```python
from build123d import *

# Parameters (mm, degrees)
F1_DEPTH = 25


with BuildPart() as f1:
    # F0 (on Top) → F1 (new body)
    with BuildSketch(Plane.XY):
        with BuildLine():
            ThreePointArc((-35.28226, -29.26819), (-33.817794, -32.803724), (-30.28226, -34.26819))
            Line((-30.28226, -34.26819), (29.71774, -34.26819))
            ThreePointArc((29.71774, -34.26819), (33.253274, -32.803724), (34.71774, -29.26819))
            Line((34.71774, -29.26819), (34.71774, -8.26819))
            ThreePointArc((34.71774, -8.26819), (31.788808, -1.197122), (24.71774, 1.73181))
            Line((24.71774, 1.73181), (-25.28226, 1.73181))
            ThreePointArc((-25.28226, 1.73181), (-32.353327, -1.197122), (-35.28226, -8.26819))
            Line((-35.28226, -8.26819), (-35.28226, -29.26819))
        make_face()
        with BuildLine():
            ThreePointArc((-16.084487, -11.432007), (-15.556147, -11.258388), (-15.011794, -11.144518))
            Line((-15.011794, -11.144518), (-15.011794, -6.116113))
            ThreePointArc((-15.011794, -6.116113), (-14.261794, -6.087948), (-13.511794, -6.116113))
            Line((-13.511794, -6.116113), (-13.511794, -11.144518))
            ThreePointArc((-13.511794, -11.144518), (-12.967699, -11.258319), (-12.439598, -11.431812))
            Line((-12.439598, -11.431812), (-9.924919, -7.077315))
            ThreePointArc((-9.924919, -7.077315), (-9.59007, -7.246285), (-9.261794, -7.427694))
            ThreePointArc((-9.261794, -7.427694), (-8.940551, -7.621285), (-8.626794, -7.826787))
            Line((-8.626794, -7.826787), (-11.140977, -12.181479))
            ThreePointArc((-11.140977, -12.181479), (-10.72626, -12.552414), (-10.355325, -12.967131))
            Line((-10.355325, -12.967131), (-6.000633, -10.452948))
            ThreePointArc((-6.000633, -10.452948), (-5.60154, -11.087948), (-5.251161, -11.751073))
            Line((-5.251161, -11.751073), (-9.605852, -14.265255))
            ThreePointArc((-9.605852, -14.265255), (-9.432234, -14.793595), (-9.318364, -15.337948))
            Line((-9.318364, -15.337948), (-4.289958, -15.337948))
            ThreePointArc((-4.289958, -15.337948), (-4.261794, -16.087948), (-4.289958, -16.837948))
            Line((-4.289958, -16.837948), (-9.318364, -16.837948))
            ThreePointArc((-9.318364, -16.837948), (-9.432235, -17.382306), (-9.605856, -17.91065))
            Line((-9.605856, -17.91065), (-5.251199, -20.424903))
            Line((-5.251199, -20.424903), (-6.000683, -21.723021))
            Line((-6.000683, -21.723021), (-10.355352, -19.2088))
            ThreePointArc((-10.355352, -19.2088), (-10.726087, -19.623309), (-11.14056, -19.994084))
            Line((-11.14056, -19.994084), (-8.626357, -24.348811))
            ThreePointArc((-8.626357, -24.348811), (-9.261794, -24.748202), (-9.925395, -25.098811))
            Line((-9.925395, -25.098811), (-12.439598, -20.744084))
            ThreePointArc((-12.439598, -20.744084), (-12.967699, -20.917577), (-13.511794, -21.031378))
            Line((-13.511794, -21.031378), (-13.511794, -26.059783))
            ThreePointArc((-13.511794, -26.059783), (-14.261794, -26.087948), (-15.011794, -26.059783))
            Line((-15.011794, -26.059783), (-15.011794, -21.031378))
            ThreePointArc((-15.011794, -21.031378), (-15.555889, -20.917577), (-16.08399, -20.744084))
            Line((-16.08399, -20.744084), (-18.598669, -25.098581))
            ThreePointArc((-18.598669, -25.098581), (-19.261794, -24.748202), (-19.896794, -24.349109))
            Line((-19.896794, -24.349109), (-17.383028, -19.994084))
            ThreePointArc((-17.383028, -19.994084), (-17.797328, -19.623482), (-18.16793, -19.209182))
            Line((-18.16793, -19.209182), (-22.522955, -21.722948))
            ThreePointArc((-22.522955, -21.722948), (-22.922048, -21.087948), (-23.272427, -20.424823))
            Line((-23.272427, -20.424823), (-18.91793, -17.910144))
            ThreePointArc((-18.91793, -17.910144), (-19.091423, -17.382043), (-19.205224, -16.837948))
            Line((-19.205224, -16.837948), (-24.233629, -16.837948))
            ThreePointArc((-24.233629, -16.837948), (-24.261794, -16.087948), (-24.233629, -15.337948))
            Line((-24.233629, -15.337948), (-19.205224, -15.337948))
            ThreePointArc((-19.205224, -15.337948), (-19.090659, -14.791005), (-18.915777, -14.260262))
            Line((-18.915777, -14.260262), (-23.298524, -11.805716))
            ThreePointArc((-23.298524, -11.805716), (-22.936977, -11.113895), (-22.522569, -10.452383))
            Line((-22.522569, -10.452383), (-18.167881, -12.966653))
            ThreePointArc((-18.167881, -12.966653), (-17.797112, -12.552198), (-17.382611, -12.181479))
            Line((-17.382611, -12.181479), (-19.896794, -7.826787))
            ThreePointArc((-19.896794, -7.826787), (-19.261794, -7.427694), (-18.598669, -7.077315))
            Line((-18.598669, -7.077315), (-16.084487, -11.432007))
        make_face(mode=Mode.SUBTRACT)
    extrude(amount=F1_DEPTH)


solid = f1.part
```
Geometry check sheet. Reference: the model listing, model coordinates, mm. A direction names the side the tool comes from. Round coordinates to 2 decimals unless told otherwise and drop trailing zeros. Order: outer loops, then holes, each group sorted by start corner. A loop starts at its lowest first (then second) coordinate and runs counter-clockwise, first axis right, second up. Notation, with made-up numbers: (-35.5, 72) - (-1.5, 72) arc R21 cw to (-1.5, 100) - close; hole circle Ø4 at (41.5, -20). An arc over 180 degrees is marked (long way). Use a Markdown table: item, result. Add a question column.
(1) Sectioned sample at A-A, the plane y = 0. Enter the section's corners in (x, z), and give its area (3 significant figures).
(2) Material ranges on line 1 along X through (y, z) = (-12, 21); line 2 along X through (y, z) = (-9.5, 3.5); line 3 along X through (y, z) = (-11, 23.25), recorded low to high. Write a range as [from, to].
(3) Release check for a two-part mould opening along X. For faces 1 (the cylindrical face through (33.214, -32.842, 12.325)), 2 (the cylindrical face through (-32.275, -1.12, 12.325)), 3 (the flat face through (-11.165, -22.952, 12.325)), 4 (the flat face through (-1, -16, 25)) record: pulls with the +X half, pulls with the -X half, needs draft (parallel to the pull), parting line crosses it, or undercut.
(4) Depth check by flat-ended pin: pin 1 (10 mm diameter, centred on y = -7.5, z = 19.5, fed in from -X). Enter the tip coordinate at first touch or a pass-through.
(5) Tool access check on faces 5 (the flat face through (0, 1.732, 12)), 6 (the flat face through (-15.012, -24, 12)). Record the directions out of +Z, -Z, +X, -X, +Y, -Y that give a thin tool (end or side, any length) a straight path to the whole face; none if there is none.
Answers below:
| question | item | result |
|---|---|---|
| 1 | outline | (-30.91, 0) - (30.34, 0) - (30.34, 25) - (-30.91, 25) - close |
| 1 | area | 1,530 mm² |
| 2 | line 1 | [-35.28, -22.95], [-19.84, -17.49], [-11.04, -8.68], [-5.68, 34.72] |
| 2 | line 2 | [-35.28, -18.93], [-17.2, -15.01], [-13.51, -11.32], [-9.59, 34.72] |
| 2 | line 3 | [-35.28, -22.87], [-21.57, -18.06], [-16.33, -15.01], [-13.51, -12.19], [-10.46, -6.95], [-5.65, 34.72] |
| 3 | face 1 | pulls with the +X half |
| 3 | face 2 | pulls with the -X half |
| 3 | face 3 | undercut |
| 3 | face 4 | needs draft |
| 4 | pin 1 | x = -35.28 |
| 5 | face 5 | +Z, -Z, +X, -X, +Y |
| 5 | face 6 | +Z, -Z |
